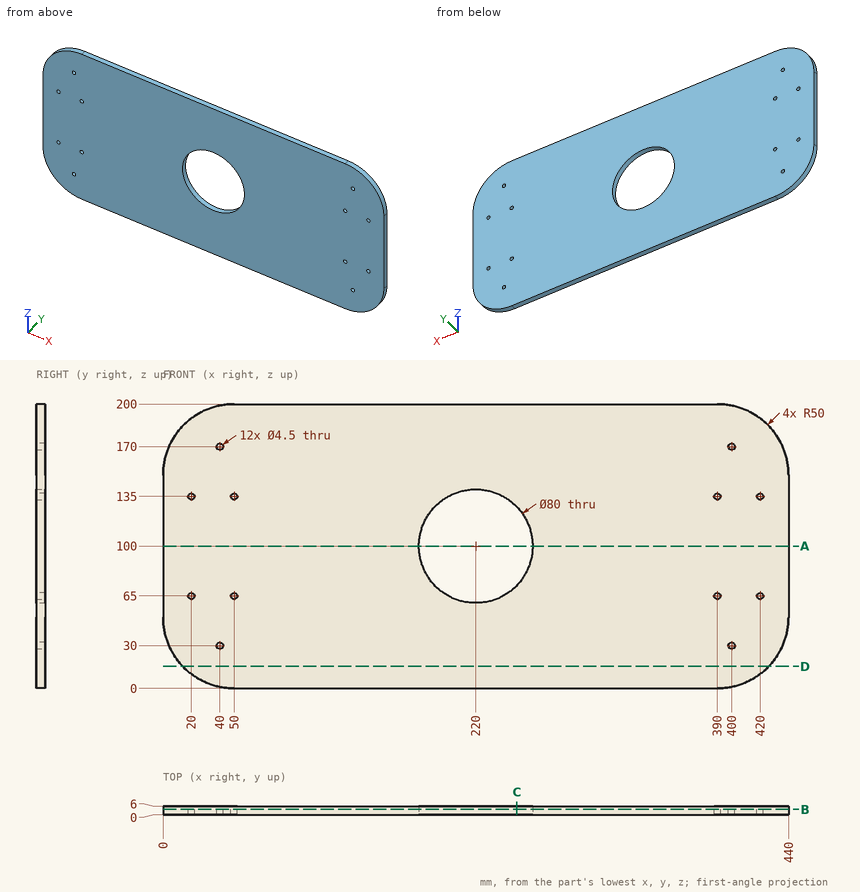
Input: dimensioned drawing with shaded views. Units: mm. Origin: part minimum x, y, z. Coordinates: 2 decimals unless noted, no trailing zeros. Order: outer loops, then holes, each group sorted by start corner. A loop starts at its lowest first (then second) coordinate and runs counter-clockwise, first axis right, second up.
1. Cut plane B-B, the plane y = 3.8. Count the separate pieces of the cut face and the enclosed holes in it, plus the area to 3 significant figures.
Checked values:
separate pieces: 1
enclosed holes: 13
area: 80,600 mm2
2. Ray query, line 1 along Z through (x, y) = (390, 3.9); line 2 along X through (y, z) = (3.6, 65); line 3 along Z through (x, y) = (40, 2.2). Return the intervals inside material, ascending.
Checked values:
line 1: z = 0 to 62.75, 67.25 to 132.75, 137.25 to 200
line 2: x = 0 to 17.75, 22.25 to 47.75, 52.25 to 200.64, 239.36 to 387.75, 392.25 to 417.75, 422.25 to 440
line 3: z = 1.01 to 27.75, 32.25 to 167.75, 172.25 to 198.99
3. Cut plane A-A, the plane z = 100. Return loops of the section in (x, y), plus the area to 3 significant figures.
Checked values:
outline: (0, 0) - (180, 0) - (180, 6) - (0, 6) - close; (260, 0) - (440, 0) - (440, 6) - (260, 6) - close
area: 2,160 mm2
4. Cut plane C-C, the plane x = 249. Return loops of the section in (y, z), plus the area to 3 significant figures.
Checked values:
outline: (0, 0) - (6, 0) - (6, 72.45) - (0, 72.45) - close; (0, 127.55) - (6, 127.55) - (6, 200) - (0, 200) - close
area: 869 mm2
5. Cut plane D-D, the plane z = 15.5. Return loops of the section in (x, y), plus the area to 3 significant figures.
Checked values:
outline: (13.81, 0) - (426.19, 0) - (426.19, 6) - (13.81, 6) - close
area: 2,470 mm2
6. Contact query for flat-ended pins moving along their axis: P1, Ø4, axis at x = 390, z = 135, coming from the -Y side; P2, Ø3, axis at y = 3.5, z = 156.5, coming from the -X side. Output: stop coordinate, or through.
Checked values:
P1: passes through
P2: stops at x = 0.25
